```python
from build123d import *

# Parameters (mm, degrees)
SKETCH1_W          = 5.98
SKETCH1_H          = 5.98
EXTRUDE1_DEPTH     = 8.6
SKETCH3_W          = 0.865
SKETCH3_H          = 0.865
EXTRUDE3_DEPTH     = 3.12
SKETCH4_R          = 1.693605641
CUT_EXTRUDE1_DEPTH = 0.254
SKETCH5_R          = 0.4826
EXTRUDE4_DEPTH     = 3.374
SKETCH6_R          = 2.99
EXTRUDE5_DEPTH     = 0.58
ESQUISSE1_R        = 2.5
BOSS_EXTRU_1_DEPTH = 7.18
SKETCH7_R          = 1.84
EXTRUDE6_DEPTH     = 6.34
SKETCH9_R          = 1.07
CUT_EXTRUDE2_DEPTH = 5.658092827
SKETCH10_R         = 0.406972167
EXTRUDE7_DEPTH     = 5.658092827
CHAMFER1_SIZE      = 0.508
CHAMFER1_SIZE2     = 0.126658625
CONG_1_R           = 0.2


with BuildPart() as part:
    # Sketch1 → Extrude1 (new body)
    with BuildSketch(Plane(origin=(0, 0, 0), x_dir=(1, 0, 0), z_dir=(0, 1, 0))):
        Rectangle(SKETCH1_W, SKETCH1_H)
    extrude(amount=EXTRUDE1_DEPTH)

    # Sketch3 → Extrude3 (add)
    with BuildSketch(Plane.XZ):
        with Locations((2.5575, 2.5575)):
            Rectangle(SKETCH3_W, SKETCH3_H)
        with Locations((2.5575, -2.5575)):
            Rectangle(SKETCH3_W, SKETCH3_H)
        with Locations((-2.5575, -2.5575)):
            Rectangle(SKETCH3_W, SKETCH3_H)
        with Locations((-2.5575, 2.5575)):
            Rectangle(SKETCH3_W, SKETCH3_H)
    extrude(amount=EXTRUDE3_DEPTH)

    # Sketch4 → Cut-Extrude1 (cut)
    with BuildSketch(Plane.XZ):
        with Locations(Location((0, 0, 0), (0, 0, 270))):
            Circle(SKETCH4_R)
    extrude(amount=-CUT_EXTRUDE1_DEPTH, mode=Mode.SUBTRACT)

    # Sketch5 → Extrude4 (add)
    with BuildSketch(Plane.XZ.offset(-0.254)):
        with Locations(Location((0, 0, 0), (0, 0, 90))):
            Circle(SKETCH5_R)
    extrude(amount=EXTRUDE4_DEPTH)

    # Sketch6 → Extrude5 (add)
    with BuildSketch(Plane.XY.offset(2.99)):
        with Locations((0, 4.9)):
            Circle(SKETCH6_R)
    extrude(amount=EXTRUDE5_DEPTH)

    # Esquisse1 → Boss.-Extru.1 (add)
    with BuildSketch(Plane.XY.offset(3.57)):
        with Locations((0, 4.9)):
            Circle(ESQUISSE1_R)
    extrude(amount=BOSS_EXTRU_1_DEPTH)

    # Sketch7 → Extrude6 (add)
    with BuildSketch(Plane.XY.offset(10.75)):
        with Locations(Location((0, 4.9, 0), (0, 0, 180))):
            Circle(SKETCH7_R)
    extrude(amount=EXTRUDE6_DEPTH)

    # Esquisse2 → Enlèvement de matière-Révolution1 (revolve, cut)
    with BuildSketch(Plane(origin=(0, 4.9, 0), x_dir=(-1, 0, 0), z_dir=(0, 1, 0)), mode=Mode.PRIVATE) as enl_vement_de_mati_re_r_volution1_sk:
        Polygon((-2.367106781, 14.512106781), (-1.66, 13.805), (-1.66, 13.475), (-2.367106781, 12.767893219), align=None)
    revolve(enl_vement_de_mati_re_r_volution1_sk.sketch.rotate(Axis((0, 4.9, 17.09), (0, 0, -1)), 180), axis=Axis((0, 4.9, 17.09), (0, 0, -1)), mode=Mode.SUBTRACT)

    # Sketch9 → Cut-Extrude2 (cut)
    with BuildSketch(Plane.XY.offset(17.09)):
        with Locations((0, 4.9)):
            Circle(SKETCH9_R)
    extrude(amount=-CUT_EXTRUDE2_DEPTH, mode=Mode.SUBTRACT)

    # Sketch10 → Extrude7 (add)
    with BuildSketch(Plane.XY.offset(11.431907173)):
        with Locations((0, 4.9)):
            Circle(SKETCH10_R)
    extrude(amount=EXTRUDE7_DEPTH)

    # Chamfer1
    chamfer1_edges = [part.edges().sort_by_distance(p)[0] for p in [
        (-0.406972167, 4.9, 17.09),
    ]]
    chamfer1_side = [part.faces().sort_by_distance(p)[0] for p in [
        (-0.406972167, 4.9, 14.260953587),
    ]]
    chamfer(chamfer1_edges, length=CHAMFER1_SIZE, length2=CHAMFER1_SIZE2, reference=chamfer1_side[0])

    # Congé1
    cong_1_edges = [part.edges().sort_by_distance(p)[0] for p in [
        (1.84, 4.9, 17.09),
        (-1.07, 4.9, 17.09),
    ]]
    fillet(cong_1_edges, radius=CONG_1_R)


solid = part.part
```
Work out the finished part from the listing and answer in its coordinate system (mm). A direction names the side the tool comes from. Give positions to 0.01 mm unless a question says otherwise; leave off trailing zeros. Order: outer loops, then holes, each group sorted by start corner. A loop starts at its lowest first (then second) coordinate and runs counter-clockwise, first axis right, second up.
1. Straight lines are drawn through the part: L1, parallel to Y at x = -0.05, z = 14.25; L2, parallel to X at y = 0.1, z = 0; L3, parallel to X at y = 5, z = 13. For each, find the intervals that lie inside material, in ascending order.
Result sheet:
L1: y = 3.06 to 3.83, 4.5 to 5.3, 5.97 to 6.74
L2: x = -2.99 to -1.69, -0.48 to 0.48, 1.69 to 2.99
L3: x = -1.84 to -1.07, -0.39 to 0.39, 1.07 to 1.84
2. The mould has two halves that part along Z. Classify faces 5 (the cylindrical face through (0.24, 3.076, 12.005)), 6 (the flat face through (0, 4, -2.99)), 7 (the cylindrical face through (0.36, 3.28, 13.64)): released by +Z, released by -Z, zero draft, split by the parting line, or undercut.
Result sheet:
face 5: zero draft
face 6: released by -Z
face 7: undercut
3. This flat-tipped pin is pushed along its axis until it touches: P1, Ø0.7, axis at x = 2.5, y = -2, coming from the +Z side. Where does it stop, or does it pass through?
Result sheet:
P1: stops at z = 2.99
4. Section B-B, the plane z = 14.75 is taken. Determine the outline of the cut face in (x, y).
Result sheet:
outline: circle Ø3.68 at (0, 4.9); circle Ø0.81 at (0, 4.9); hole circle Ø2.14 at (0, 4.9)
5. Section D-D, the plane z = 4.5 is taken. Determine the outline of the cut face in (x, y), and give its area (3 significant figures).
Result sheet:
outline: circle Ø5 at (0, 4.9)
area: 19.6 mm2
6. Section A-A, the plane y = -1.75 is taken. Determine the outline of the cut face in (x, z) (3 decimals), and give its area (3 significant figures).
Result sheet:
outline: (-2.99, -2.99) - (-2.125, -2.99) - (-2.125, -2.125) - (-2.99, -2.125) - close; (-2.99, 2.125) - (-2.125, 2.125) - (-2.125, 2.99) - (-2.99, 2.99) - close; circle Ø0.965 at (0, 0); (2.125, -2.99) - (2.99, -2.99) - (2.99, -2.125) - (2.125, -2.125) - close; (2.125, 2.125) - (2.99, 2.125) - (2.99, 2.99) - (2.125, 2.99) - close
area: 3.72 mm2
7. For faces 1 (the flat face through (2.6, -1.5, 2.125)), 2 (the flat face through (-1, 0.254, 0)), 3 (the cylindrical face through (0.24, 3.076, 15.417)), 4 (the flat face through (2.99, 4, 0)), determine the directions among +Z, -Z, +X, -X, +Y, -Y from which every point of the face is accessible in a straight line to the end or side of a thin tool.
Result sheet:
face 1: +X, -X, -Y
face 2: -Y
face 3: +Z
face 4: +Z, -Z, +X, +Y, -Y
8. Section C-C, the plane z = 0 is taken. Determine the outline of the cut face in (x, y).
Result sheet:
outline: (-2.99, 0) - (-1.69, 0) - (-1.69, 0.25) - (-0.48, 0.25) - (-0.48, -3.12) - (0.48, -3.12) - (0.48, 0.25) - (1.69, 0.25) - (1.69, 0) - (2.99, 0) - (2.99, 8.6) - (-2.99, 8.6) - close
